from build123d import *

# Parameters (mm, degrees)
SWEEP_THIN3_PROFILE_R   = 15
SWEEP_THIN3_PROFILE_R_2 = 13
SKETCH57_W              = 35
SKETCH57_H              = 35
BOSS_EXTRUDE1_DEPTH     = 8
SKETCH58_W              = 35
SKETCH58_H              = 8
BOSS_EXTRUDE2_DEPTH     = 40
FILLET1_R               = 17.5
SKETCH59_R              = 5
CUT_EXTRUDE1_DEPTH      = 549.85107275
SKETCH60_W              = 35
SKETCH60_H              = 8
BOSS_EXTRUDE3_DEPTH     = 55
FILLET2_R               = 17.5
SKETCH61_R              = 5
CUT_EXTRUDE2_DEPTH      = 55
FILLET2_OF_MIRROR1_R    = 17.5


with BuildPart() as part:
    # Sweep-Thin3: sweep along a path in Sketch44
    with BuildLine(Plane.XY) as sweep_thin3_path:
        Line((0, 0), (200, 0))
        ThreePointArc((200, 0), (256.568542495, 23.431457505), (280, 80))
        Line((280, 80), (280, 480))
    # Sweep-Thin3 profile (on start of the path) → Sweep-Thin3 (sweep)
    with BuildSketch(Plane(origin=(0, 0, 0), x_dir=(0, 0, 1), z_dir=(1, 0, 0))):
        Circle(SWEEP_THIN3_PROFILE_R)
        Circle(SWEEP_THIN3_PROFILE_R_2, mode=Mode.SUBTRACT)
    sweep(path=sweep_thin3_path.line)

    # Sketch57 → Boss-Extrude1 (add)
    with BuildSketch(Plane.ZY):
        Rectangle(SKETCH57_W, SKETCH57_H)
    extrude(amount=BOSS_EXTRUDE1_DEPTH)

    # Sketch58 → Boss-Extrude2 (add)
    with BuildSketch(Plane.ZY.offset(8)):
        with Locations((0, 13.5)):
            Rectangle(SKETCH58_W, SKETCH58_H)
        with Locations((0, -13.5)):
            Rectangle(SKETCH58_W, SKETCH58_H)
    extrude(amount=BOSS_EXTRUDE2_DEPTH)

    # Fillet1
    fillet1_edges = [part.edges().sort_by_distance(p)[0] for p in [
        (-48, -13.5, 17.5),
        (-48, -13.5, -17.5),
        (-48, 13.5, 17.5),
        (-48, 13.5, -17.5),
    ]]
    fillet(fillet1_edges, radius=FILLET1_R - 0.0001)  # a hair under: the kernel refuses the full size

    # Sketch59 → Cut-Extrude1 (cut, through all)
    with BuildSketch(Plane(origin=(0, 17.5, 0), x_dir=(1, 0, 0), z_dir=(0, 1, 0))):
        with Locations(Location((-30.5, 0, 0), (0, 0, 270))):
            Circle(SKETCH59_R)
    extrude(amount=-CUT_EXTRUDE1_DEPTH, mode=Mode.SUBTRACT)

    # Sketch60 → Boss-Extrude3 (add)
    with BuildSketch(Plane.XY):
        with Locations((150, 0)):
            Rectangle(SKETCH60_W, SKETCH60_H)
    boss_extrude3 = extrude(amount=BOSS_EXTRUDE3_DEPTH)

    # Fillet2
    fillet2_edges = [part.edges().sort_by_distance(p)[0] for p in [
        (132.5, 0, 55),
        (167.5, 0, 55),
    ]]
    fillet(fillet2_edges, radius=FILLET2_R - 0.0001)  # a hair under: the kernel refuses the full size

    # Sketch61 → Cut-Extrude2 (cut)
    with BuildSketch(Plane(origin=(0, 4, 0), x_dir=(1, 0, 0), z_dir=(0, 1, 0))):
        with Locations(Location((150, -37.5, 0), (0, 0, 180))):
            Circle(SKETCH61_R)
    cut_extrude2 = extrude(amount=-CUT_EXTRUDE2_DEPTH, mode=Mode.SUBTRACT)

    # Mirror1: Boss-Extrude3, Cut-Extrude2 across plane
    add(boss_extrude3.mirror(Plane.XY))
    add(cut_extrude2.mirror(Plane.XY), mode=Mode.SUBTRACT)

    # Fillet2 of Mirror1
    fillet2_of_mirror1_edges = [part.edges().sort_by_distance(p)[0] for p in [
        (132.5, 0, -55),
        (167.5, 0, -55),
    ]]
    fillet(fillet2_of_mirror1_edges, radius=FILLET2_OF_MIRROR1_R - 0.0001)  # a hair under: the kernel refuses the full size


solid = part.part
Part model, mm, in its own coordinate system. A direction names the side the tool comes from. Coordinates: 2 decimals unless noted, no trailing zeros. Loops run counter-clockwise (first coordinate to the right, second up) from the corner with the lowest first, then second, coordinate; pieces in that order, holes last. Notation, with made-up numbers: M 44,57 L 74,57 A14 cw 74,63 Z; hole C -21.5,65.5 d1. An arc over 180 degrees is marked long. Use a Markdown table: item, result. Add a question column.
Q1. Cut at B-B (y = 266). Write the cut outline in (x, z).
Q2. Which spindle directions (+Z, -Z, +X, -X, +Y, -Y) get a long thin tool onto all of the face, cutting with end or side? Do faces 5 (the cylindrical face through (267.31, 282.8, -2.82)), 6 (the flat face through (-24, 17.5, 0)), 7 (the flat face through (150, -4, -30)), 8 (the flat face through (-23, 9.5, 0)), 9 (the flat face through (0, 0, 0)). Say none if no direction does.
Q3. Mould opens along Y. For faces 1 (the cylindrical face through (101.4, 12.69, -2.82)), 2 (the cylindrical face through (101.4, 5.745, 13.856)), 3 (the flat face through (150, 4, 0)), 4 (the cylindrical face through (162.51, 0.06, -49.74)) say: +Y half, -Y half, draft (parallel to the pull), parting line (faces both ways), or undercut.
Q4. Pin check, flat tips, straight feed: P1, Ø8, axis at x = -30.5, z = 0, coming from the +Y side; P2, Ø10.5, axis at x = 157, z = -28, coming from the +Y side; P3, Ø9, axis at y = -1.5, z = -28, coming from the -X side; P4, Ø5.5, axis at y = -3, z = -4.5, coming from the -X side. Stop position of each tip, or through.
Q5. Cut at A-A (x = 5.5). Write the cut outline in (y, z).
Q6. Probe L1, parallel to Z at x = 150, y = -1.5; L2, parallel to Y at x = 83, z = -4; L3, parallel to X at y = 279, z = 10. List the from-to ranges inside material, lowest first.
Worked out:
| question | item | result |
|---|---|---|
| 1 | outline | C 280,0 d30; hole C 280,0 d26 |
| 2 | face 5 | +Y |
| 2 | face 6 | +Z, -Z, -X, +Y |
| 2 | face 7 | -Z, +X, -Y |
| 2 | face 8 | +Z, -Z, -X |
| 2 | face 9 | none |
| 3 | face 1 | undercut |
| 3 | face 2 | parting line |
| 3 | face 3 | undercut |
| 3 | face 4 | draft |
| 4 | P1 | passes through |
| 4 | P2 | stops at y = 4 |
| 4 | P3 | stops at x = 132.5 |
| 4 | P4 | stops at x = -8 |
| 5 | outline | C 0,0 d30; hole C 0,0 d26 |
| 6 | L1 | z = -55 to -42.5, -32.5 to 32.5, 42.5 to 55 |
| 6 | L2 | y = -14.46 to -12.37, 12.37 to 14.46 |
| 6 | L3 | x = 268.82 to 271.69, 288.31 to 291.18 |
